```python
from build123d import *

# Parameters (mm, degrees)
SKETCH1_W           = 20
SKETCH1_H           = 10
BOSS_EXTRUDE1_DEPTH = 3
SKETCH2_W           = 9.8
SKETCH2_H           = 8.5
SKETCH2_W_2         = 5.8
SKETCH2_H_2         = 4.5
BOSS_EXTRUDE2_DEPTH = 3
BOSS_EXTRUDE3_DEPTH = 1


with BuildPart() as part:
    # Sketch1 → Boss-Extrude1 (new body)
    with BuildSketch(Plane(origin=(0, 0, 0), x_dir=(1, 0, 0), z_dir=(0, 1, 0))):
        Rectangle(SKETCH1_W, SKETCH1_H)
    extrude(amount=BOSS_EXTRUDE1_DEPTH)

    # Sketch2 → Boss-Extrude2 (add)
    with BuildSketch(Plane.XZ):
        Rectangle(SKETCH2_W, SKETCH2_H)
        Rectangle(SKETCH2_W_2, SKETCH2_H_2, mode=Mode.SUBTRACT)
    extrude(amount=BOSS_EXTRUDE2_DEPTH)

    # Sketch3 → Boss-Extrude3 (add)
    with BuildSketch(Plane(origin=(0, 3, 0), x_dir=(1, 0, 0), z_dir=(0, 1, 0))):
        Polygon((-8.215384615, -2.5), (-7.555328526, 2.5), (-7.491225962, 2.5), (-5.426923077, -1.602564103), (-3.367628205, 2.5), (-3.302524038, 2.5), (-2.638461538, -2.5), (-3.089182692, -2.5), (-3.567948718, 1.09775641), (-5.372836538, -2.5), (-5.473998397, -2.5), (-7.285897436, 1.105769231), (-7.763661859, -2.5), align=None)
        with BuildLine():
            Line((-1.612820513, 2.5), (-1.164102564, 2.5))
            Line((-1.164102564, 2.5), (-1.164102564, -0.495793269))
            add(Edge.make_bspline(
                [(-1.164102564, -0.495793269), (-1.164169341, -0.53819432), (-1.164296062, -0.618657622), (-1.163449614, -0.733183765), (-1.161079088, -0.835001564), (-1.159584574, -0.924503489), (-1.156259812, -1.001278843), (-1.153548316, -1.065743572), (-1.150061807, -1.117592433), (-1.145871639, -1.147850899), (-1.144070513, -1.160857372)],
                knots=[0, 0, 0, 0, 1.528628734, 2.90083645, 4.128790002, 5.200304208, 6.127813768, 6.898992206, 7.526736466, 8, 8, 8, 8], degree=3))
            add(Edge.make_bspline(
                [(-1.144070513, -1.160857372), (-1.136674143, -1.207781319), (-1.122298163, -1.298985218), (-1.08566048, -1.428854192), (-1.034492622, -1.545899133), (-0.973859703, -1.653772406), (-0.893955973, -1.749471491), (-0.798236637, -1.837630995), (-0.682268396, -1.914733574), (-0.553324674, -1.985234733), (-0.414345763, -2.041899137), (-0.272329668, -2.0847468), (-0.129411126, -2.110859514), (-0.033730891, -2.113883141), (0.013782051, -2.115384615)],
                knots=[0, 0, 0, 0, 1.035780045, 2.013197591, 2.933192213, 3.817615948, 4.702609284, 5.640816605, 6.646850145, 7.73207398, 8.84249596, 9.914020372, 10.964143139, 12, 12, 12, 12], degree=3))
            add(Edge.make_bspline(
                [(0.013782051, -2.115384615), (0.054573109, -2.113850544), (0.135919626, -2.11079126), (0.256785956, -2.091846359), (0.374500396, -2.057702694), (0.489644225, -2.013645896), (0.597574203, -1.955435051), (0.698350548, -1.888190995), (0.788299026, -1.809318315), (0.87038188, -1.722032109), (0.94186036, -1.62354668), (1.003819133, -1.516006483), (1.054570461, -1.39779313), (1.07963264, -1.314715384), (1.092508013, -1.272035256)],
                knots=[0, 0, 0, 0, 0.994687771, 1.983630487, 2.973142513, 3.978332533, 4.983357753, 5.956394766, 6.925816176, 7.893390482, 8.871859704, 9.88551698, 10.913711441, 12, 12, 12, 12], degree=3))
            add(Edge.make_bspline(
                [(1.092508013, -1.272035256), (1.096793906, -1.254394436), (1.106344604, -1.215083579), (1.115268954, -1.148624592), (1.12456399, -1.070211215), (1.131013376, -0.979280054), (1.137300833, -0.876135807), (1.141062366, -0.760241154), (1.142800984, -0.632016924), (1.143319099, -0.542535264), (1.143589744, -0.495793269)],
                knots=[0, 0, 0, 0, 0.558680831, 1.244966039, 2.062412453, 2.990489873, 4.051219941, 5.244515665, 6.560634259, 8, 8, 8, 8], degree=3))
            Line((1.143589744, -0.495793269), (1.143589744, 2.5))
            Line((1.143589744, 2.5), (1.592307692, 2.5))
            Line((1.592307692, 2.5), (1.592307692, -0.519831731))
            add(Edge.make_bspline(
                [(1.592307692, -0.519831731), (1.591944663, -0.574257986), (1.59123619, -0.680474133), (1.585092509, -0.836118932), (1.575296795, -0.983766048), (1.561456669, -1.123435329), (1.543118093, -1.254626985), (1.522724921, -1.37849094), (1.49675416, -1.494138072), (1.466420729, -1.602470097), (1.431744232, -1.705592259), (1.386828306, -1.803461709), (1.336221878, -1.899053708), (1.276200945, -1.990922435), (1.208756112, -2.079474654), (1.132396569, -2.164173332), (1.049647767, -2.24637197), (0.959134111, -2.323962064), (0.862347646, -2.395117317), (0.759576278, -2.457685562), (0.651609464, -2.510576444), (0.538727855, -2.554113479), (0.42088328, -2.58684862), (0.298072766, -2.6112417), (0.170016775, -2.625102125), (0.082924409, -2.627162025), (0.038822115, -2.628205128)],
                knots=[0, 0, 0, 0, 1.316592851, 2.569410997, 3.76748051, 4.895814652, 5.963796859, 6.97159953, 7.931736103, 8.829262218, 9.692595152, 10.560224239, 11.431080259, 12.30701507, 13.211635791, 14.121146779, 15.063487852, 16.031507147, 17.00238618, 17.966455255, 18.938106653, 19.907068911, 20.888905087, 21.893141452, 22.933117798, 24, 24, 24, 24], degree=3))
            add(Edge.make_bspline(
                [(0.038822115, -2.628205128), (-0.009276603, -2.627084035), (-0.103646115, -2.624884454), (-0.242700497, -2.612280525), (-0.376006492, -2.588539962), (-0.50497203, -2.558311471), (-0.627841312, -2.516620418), (-0.746260518, -2.467908811), (-0.858201491, -2.408084153), (-0.965480247, -2.341522163), (-1.065229898, -2.266629823), (-1.156797617, -2.185001003), (-1.240334575, -2.097943321), (-1.314432713, -2.004514227), (-1.380319691, -1.90544036), (-1.437077138, -1.800441446), (-1.485810344, -1.689558137), (-1.510962583, -1.612482137), (-1.523677885, -1.573517628)],
                knots=[0, 0, 0, 0, 1.13879206, 2.234305948, 3.301075583, 4.341971843, 5.366689343, 6.369221514, 7.369726634, 8.367512178, 9.355451585, 10.318319045, 11.268648973, 12.207971039, 13.137398894, 14.081662264, 15.030215811, 16, 16, 16, 16], degree=3))
            add(Edge.make_bspline(
                [(-1.523677885, -1.573517628), (-1.531073825, -1.546899665), (-1.547115784, -1.489164709), (-1.564294781, -1.393612583), (-1.578736326, -1.283591272), (-1.592315695, -1.159093245), (-1.600328492, -1.020022007), (-1.607353404, -0.866437842), (-1.612870002, -0.698155039), (-1.61283747, -0.580934303), (-1.612820513, -0.519831731)],
                knots=[0, 0, 0, 0, 0.625038921, 1.35572334, 2.194682327, 3.136881307, 4.189498639, 5.346923369, 6.617055217, 8, 8, 8, 8], degree=3))
            Line((-1.612820513, -0.519831731), (-1.612820513, 2.5))
        make_face()
        Polygon((2.297435897, 1.987179487), (2.297435897, 2.5), (4.925641026, 2.5), (4.925641026, 1.987179487), (3.835897436, 1.987179487), (3.835897436, -2.5), (3.387179487, -2.5), (3.387179487, 1.987179487), align=None)
        Polygon((5.694871795, 2.5), (8.515384615, 2.5), (8.515384615, 1.987179487), (6.143589744, 1.987179487), (6.143589744, 0.448717949), (8.515384615, 0.448717949), (8.515384615, -0.064102564), (6.143589744, -0.064102564), (6.143589744, -1.987179487), (8.515384615, -1.987179487), (8.515384615, -2.5), (5.694871795, -2.5), align=None)
    extrude(amount=BOSS_EXTRUDE3_DEPTH)


solid = part.part
```
Geometry check sheet. Reference: the model listing, model coordinates, mm. A direction names the side the tool comes from. Round coordinates to 2 decimals unless told otherwise and drop trailing zeros. Order: outer loops, then holes, each group sorted by start corner. A loop starts at its lowest first (then second) coordinate and runs counter-clockwise, first axis right, second up. Notation, with made-up numbers: (9, 67.5) -> (26, 67.5) arc R14 ccw to (26, 76.5) -> close; hole circle Ø9 at (-39.5, 64). An arc over 180 degrees is marked (long way). Return JSON: item names as keys, results as strings. Group by question number.
Q1. Tool access check on faces 5 (the flat face through (7.3, 3.5, -0.449)), 6 (the flat face through (0, 0, 0)), 7 (the flat face through (0, -1, -4.25)), 8 (the flat face through (-3.325, 3.493, 0.726)), 9 (the flat face through (-2.975, 3.493, -0.035)). Record the directions out of +Z, -Z, +X, -X, +Y, -Y that give a thin tool (end or side, any length) a straight path to the whole face; none if there is none.
Q2. Section check A-A, the plane x = 7.25. Record the boundary of the cut face in (y, z).
Q3. Section check C-C, the plane z = 3.25. Record the boundary of the cut face in (x, y).
Q4. Section check B-B, the plane y = -0.25. Record the boundary of the cut face in (x, z).
Q5. Material ranges on probe 1 along Z at (x, y) = (2, -2.5); probe 2 along X at (y, z) = (-1, -2); probe 3 along Y at (x, z) = (-4.5, 4.75), recorded low to high. Write a range as from..to.
Q6. Gauge pin test, flat ends, axial feed: pin 1 (0.5 mm diameter, centred on x = 3, y = 3.5, fed in from +Z); pin 2 (0.5 mm diameter, centred on x = 7.5, y = 3.5, fed in from +Z); pin 3 (0.5 mm diameter, centred on x = 7.5, y = 3.5, fed in from -Z). Record the tip position at first contact, or that the pin passes through.
Q7. Release check for a two-part mould opening along Z. For faces 1 (the flat face through (-7.52, 3.49, 0.67)), 2 (the flat face through (-4.41, 3.49, -0.42)), 3 (the flat face through (3.6, 4, -0.6)), 4 (the flat face through (0, -1, 2.25)) record: released by +Z, released by -Z, zero draft, split by the parting line, or undercut.
Q8. Section check D-D, the plane x = 2.5. Record the boundary of the cut face in (y, z).
Numbers:
{
 "1": {"face 5": "+X, +Y", "face 6": "-Y", "face 7": "-Z, +X, -X, -Y", "face 8": "+Z, +Y", "face 9": "-Z, +Y"},
 "2": {"outline": "(0, -5) -> (3, -5) -> (3, -2.5) -> (4, -2.5) -> (4, -1.99) -> (3, -1.99) -> (3, -0.45) -> (4, -0.45) -> (4, 0.06) -> (3, 0.06) -> (3, 1.99) -> (4, 1.99) -> (4, 2.5) -> (3, 2.5) -> (3, 5) -> (0, 5) -> close"},
 "3": {"outline": "(-10, 0) -> (-4.9, 0) -> (-4.9, -3) -> (4.9, -3) -> (4.9, 0) -> (10, 0) -> (10, 3) -> (-10, 3) -> close"},
 "4": {"outline": "(-4.9, -4.25) -> (4.9, -4.25) -> (4.9, 4.25) -> (-4.9, 4.25) -> close; hole (-2.9, -2.25) -> (2.9, -2.25) -> (2.9, 2.25) -> (-2.9, 2.25) -> close"},
 "5": {"probe 1": "-4.25..-2.25, 2.25..4.25", "probe 2": "-4.9..-2.9, 2.9..4.9", "probe 3": "0..3"},
 "6": {"pin 1": "z = -1.99", "pin 2": "z = 2.5", "pin 3": "z = -2.5"},
 "7": {"face 1": "released by +Z", "face 2": "released by -Z", "face 3": "zero draft", "face 4": "undercut"},
 "8": {"outline": "(-3, -4.25) -> (0, -4.25) -> (0, -5) -> (3, -5) -> (3, -2.5) -> (4, -2.5) -> (4, -1.99) -> (3, -1.99) -> (3, 5) -> (0, 5) -> (0, 4.25) -> (-3, 4.25) -> (-3, 2.25) -> (0, 2.25) -> (0, -2.25) -> (-3, -2.25) -> close"}
}
